```python
from build123d import *

# Parameters (mm, degrees)
SKETCH_1_W               = 1000
SKETCH_1_H               = 700
EXTRUDE_1_DEPTH          = 200
SKETCH_2_R               = 100
EXTRUDE_2_DEPTH          = 100
MIRROR_2_COPY_1_SKETCH_R = 100
MIRROR_2_COPY_1_DEPTH    = 100
SKETCH_3_W               = 608.816937559
SKETCH_3_H               = 534.376438644
CUT_EXTRUDE_1_DEPTH      = 83
CUT_EXTRUDE_1_DRAFT      = -20


with BuildPart() as part:
    # 草图1 → 凸台-拉伸1 (new body)
    with BuildSketch(Plane(origin=(0, 0, 0), x_dir=(1, 0, 0), z_dir=(0, 1, 0))):
        Rectangle(SKETCH_1_W, SKETCH_1_H)
    extrude(amount=EXTRUDE_1_DEPTH)

    # 草图2 → 凸台-拉伸2 (add)
    with BuildSketch(Plane.XY.offset(350)):
        with Locations((-500, 0)):
            Circle(SKETCH_2_R)
    extrude_2 = extrude(amount=EXTRUDE_2_DEPTH)

    # 镜向1: 凸台-拉伸2 across plane
    add(extrude_2.mirror(Plane(origin=(0, 0, 0), x_dir=(0, 0, 1), z_dir=(1, 0, 0))))

    # 镜向2: 凸台-拉伸2 across plane
    add(extrude_2.mirror(Plane.XY))

    # 镜向2 copy 1 sketch → 镜向2 copy 1 (add)
    with BuildSketch(Plane(origin=(0, 0, -350), x_dir=(-1, 0, 0), z_dir=(0, 0, -1))):
        with Locations((-500, 0)):
            Circle(MIRROR_2_COPY_1_SKETCH_R)
    extrude(amount=MIRROR_2_COPY_1_DEPTH)


with BuildPart() as cut_extrude_1_tool:
    # 草图3 → 切除-拉伸1 (with draft: the straight prism first)
    with BuildSketch(Plane(origin=(0, 200, 0), x_dir=(1, 0, 0), z_dir=(0, 1, 0))):
        with Locations((120.965810738, 0)):
            Rectangle(SKETCH_3_W, SKETCH_3_H)
    extrude(amount=-CUT_EXTRUDE_1_DEPTH)
    # 切除-拉伸1: the draft: its side faces are tilted about the plane it starts from
    cut_extrude_1_sides = [cut_extrude_1_tool.faces().sort_by_distance(p)[0] for p in [
        (120.965810738, 158.5, 267.188219322),
        (425.374279517, 158.5, 0),
        (120.965810738, 158.5, -267.188219322),
        (-183.442658042, 158.5, 0),
    ]]
    draft(cut_extrude_1_sides, Plane(origin=(0, 200, 0), x_dir=(1, 0, 0), z_dir=(0, 1, 0)), CUT_EXTRUDE_1_DRAFT)


with BuildPart() as part_1:
    add(part.part)

    # 切除-拉伸1: cut by cut_extrude_1_tool
    add(cut_extrude_1_tool.part, mode=Mode.SUBTRACT)


solid = part_1.part
```
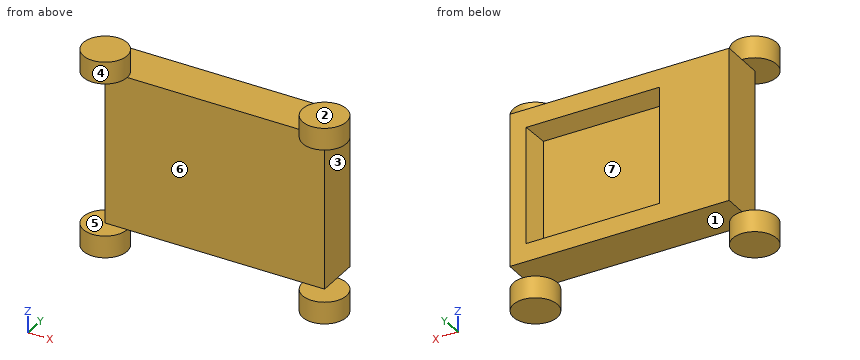
Work out the finished part from the listing and answer in its coordinate system (mm). Face numbers are marked on the shaded views. A direction names the side the tool comes from. Give positions to 0.01 mm unless a question says otherwise; leave off trailing zeros. Loops run counter-clockwise (first coordinate to the right, second up) from the corner with the lowest first, then second, coordinate; pieces in that order, holes last. Notation, with made-up numbers: M 44,31 L 48,31 A35 ccw 48,63 Z; hole C 45.25,55.5 d1. An arc over 180 degrees is marked long. One line per item, written item: value. Start each with the question number.
1. Find section A-A (x = 190). Give the vertices of the cut face in (y, z), and give its area (3 significant figures).
2. Find section B-B (y = -15.5). Give the vertices of the cut face in (x, z), and give its area (3 significant figures).
3. Which of the six approach directions +Z, -Z, +X, -X, +Y, -Y give full straight-line access (tool end or side, diameter ignored) to the marked faces 4, 5, 6 and 7?
4. Find the intervals of material crossed by probe 1 along Z at (x, y) = (495.5, -82); probe 2 along X at (y, z) = (-0.5, -409); probe 3 along Y at (x, z) = (108, -182.5), in increasing order.
5. Find section C-C (y = 138). Give the vertices of the cut face in (x, z).
6. Find section D-D (x = -443.5). Give the vertices of the cut face in (y, z).
7. Determine the mould class of the marked faces 1, 2 and 3 for opening direction Z: released by +Z, released by -Z, zero draft, split by the parting line, or undercut.
8. Each of these flat-tipped pins is pushed along its axis until it touches: P1, Ø4, axis at x = -156, z = -99.5, coming from the -Y side; P2, Ø1.5, axis at x = 173, z = 134, coming from the +Y side; P3, Ø1.5, axis at y = 1, z = 216, coming from the +X side. Where does it stop, or does it pass through?
Reported:
1. outline: M 0,-350 L 200,-350 L 200,-267.19 L 117,-236.98 L 117,236.98 L 200,267.19 L 200,350 L 0,350 Z
1. area: 98,200 mm²
2. outline: M -598.79,-450 L -401.21,-450 L -401.21,-350 L -598.79,-350 Z; M -598.79,350 L -401.21,350 L -401.21,450 L -598.79,450 Z; M 401.21,-450 L 598.79,-450 L 598.79,-350 L 401.21,-350 Z; M 401.21,350 L 598.79,350 L 598.79,450 L 401.21,450 Z
2. area: 79,000 mm²
3. face 4: +Z
3. face 5: -X, -Y
3. face 6: +X, -X, -Y
3. face 7: +Y
4. probe 1: z = -450 to -350, 350 to 450
4. probe 2: x = -600 to -400, 400 to 600
4. probe 3: y = 0 to 117
5. outline: M -500,-350 L 500,-350 L 500,350 L -500,350 Z; hole M -160.88,-244.62 L 402.81,-244.62 L 402.81,244.62 L -160.88,244.62 Z
6. outline: M -82.51,-450 L 82.51,-450 L 82.51,-350 L 200,-350 L 200,350 L 82.51,350 L 82.51,450 L -82.51,450 L -82.51,350 L 0,350 L 0,-350 L -82.51,-350 Z
7. face 1: released by -Z
7. face 2: released by +Z
7. face 3: undercut
8. P1: stops at y = 0
8. P2: stops at y = 117
8. P3: stops at x = 500
